Autodesk Inventor part; units mm, degrees
ref_plane "YZ Plane" through (0, 0, 0) normal (1, 0, 0) x (0, 1, 0)
ref_plane "XZ Plane" through (0, 0, 0) normal (0, 1, 0) x (-1, 0, 0)
ref_plane "XY Plane" through (0, 0, 0) normal (0, 0, 1) x (1, 0, 0)
sketch "Sketch1" plane through (0, 0, 0) normal (0, 0, 1) x (1, 0, 0)
  line L0 (-11.8297, 9.3175) -> (-7.8297, 9.3175)
  line L1 (-7.8297, 9.3175) -> (-7.8297, -24.6825)
  line L2 (-11.8297, -24.6825) -> (-11.8297, 9.3175)
  line L3 (16.1703, -24.6825) -> (16.1703, -28.6825)
  line L4 (16.1703, -28.6825) -> (-11.8297, -28.6825)
  line L5 (-11.8297, -28.6825) -> (-11.8297, -24.6825)
  line L6 (12.1703, -24.6825) -> (12.1703, 9.3175)
  line L7 (12.1703, 9.3175) -> (16.1703, 9.3175)
  line L8 (16.1703, 9.3175) -> (16.1703, -24.6825)
  line L9 (12.1703, -24.6825) -> (-7.8297, -24.6825)
  point P0 (0, 0)
  dimension "d0" = 4
  dimension "d1" = 34
  dimension "d5" = 4
  dimension "d6" = 4
  dimension "d7" = 34
  dimension "d14" = 24
  dimension "d15" = 28
  dimension "d16" = 38
  dimension "d18" = 9.3175
extrude "Extrusion1" add sketch "Sketch1" along normal blind 30
sketch "Sketch2" plane through (-11.8297, -28.6825, 0) normal (-1, 0, 0) x (0, 0, 1)
  line L0 (0, 0) -> (0, 38) construction
  line L1 (0, 0) -> (30, 0) construction
  line L2 (30, 38) -> (30, 0) construction
  line L3 (0, 38) -> (30, 38) construction
  line L4 (0, 38) -> (30, 38) construction
  line L5 (15, 38) -> (15, 0) construction
  circle A0 centre (15, 29.8727) radius 3.25
  point P0 (0, 28.6825)
  dimension "d10" = 6.5
extrude "Extrusion2" cut sketch "Sketch2" against normal through all
fillet "Fillet1" radius 10 4 edges at (-9.8297, 9.3175, 0) (14.1703, 9.3175, 0) (-9.8297, 9.3175, 30) (14.1703, 9.3175, 30)
sketch "Sketch3" plane through (-7.8297, -24.6825, 0) normal (0, 1, 0) x (1, 0, 0)
  line L0 (0, 0) -> (20, 0)
  line L1 (0, 0) -> (0, -30)
  line L2 (20, -30) -> (0, -30)
  line L3 (20, 0) -> (20, -30)
  circle A0 centre (10, -15) radius 4.25
  point P0 (7.8297, 0)
  dimension "d19" = 8.5
extrude "Extrusion3" cut sketch "Sketch3" against normal through all contours A0
fillet "Fillet2" radius 2 2 edges at (-7.8297, -24.6825, 15) (12.1703, -24.6825, 15)
equation "\"d1\" = d7"
properties part number "linear actuator bracket"
Check sheet for the modelled part. Datum: model origin and axes. Units: mm. A direction names the side the tool comes from. Give positions to 0.01 mm unless a question says otherwise; leave off trailing zeros. Loops run counter-clockwise (first coordinate to the right, second up) from the corner with the lowest first, then second, coordinate; pieces in that order, holes last. Notation, with made-up numbers: M -18,-25 L 24,-25 A18 cw 24,5 Z; hole C 33,80.25 d4. An arc over 180 degrees is marked long. Use a Markdown table: item, result. Add a question column.
Q1. Sectioned sample at D-D, the plane y = 3. Record the cut outline in (x, z).
Q2. Go/stop test with a flat-tipped pin: pin 1 (5 mm diameter, centred on y = 1.19, z = 15, fed in from -X). Record where the tip stops, or that it passes through.
Q3. Tool access check on faces 1 (the flat face through (-7.83, -6, 15)), 2 (the cylindrical face through (14.2, 6.47, 26.99)). Record the directions out of +Z, -Z, +X, -X, +Y, -Y that give a thin tool (end or side, any length) a straight path to the whole face; none if there is none.
Q4. Sectioned sample at C-C, the plane x = 0.5. Record the cut outline in (y, z), then the cut area to 3 significant figures.
Q5. Mould release check, pull along Z, two halves, no side actions. Record for faces 3 (the flat face through (2, -25, 30)), 4 (the cylindrical face through (14.2, 6.31, 2.85)), 5 (the cylindrical face through (-9.858, 1.333, 11.753)), 6 (the flat face through (5.5, -28.682, 18.1)): pulls with the +Z half, pulls with the -Z half, needs draft (parallel to the pull), parting line crosses it, or undercut.
Q6. Sectioned sample at B-B, the plane z = 15. Record the cut outline in (x, y), then the cut area to 3 significant figures.
Q7. Sectioned sample at A-A, the plane y = -12. Record the cut outline in (x, z).
Q8. Scan lines: line 1 along X through (y, z) = (6, 14.25); line 2 along X through (y, z) = (-26.45, 15); line 3 along Y through (x, z) = (13.05, 15). Record each from-to range of solid material in increasing order. Write a range as [from, to].
Verdict:
| question | item | result |
|---|---|---|
| 1 | outline | M -11.83,0.7 L -7.83,0.7 L -7.83,12.3 L -11.83,12.3 Z; M -11.83,17.7 L -7.83,17.7 L -7.83,29.3 L -11.83,29.3 Z; M 12.17,0.7 L 16.17,0.7 L 16.17,12.3 L 12.17,12.3 Z; M 12.17,17.7 L 16.17,17.7 L 16.17,29.3 L 12.17,29.3 Z |
| 2 | pin 1 | through |
| 3 | face 1 | +Z, -Z, +Y |
| 3 | face 2 | +Z, +X, -X, +Y |
| 4 | outline | M -28.68,0 L -24.68,0 L -24.68,11.09 L -28.68,11.09 Z; M -28.68,18.91 L -24.68,18.91 L -24.68,30 L -28.68,30 Z |
| 4 | area | 88.7 mm^2 |
| 5 | face 3 | pulls with the +Z half |
| 5 | face 4 | pulls with the -Z half |
| 5 | face 5 | undercut |
| 5 | face 6 | needs draft |
| 6 | outline | M -11.83,-28.68 L -2.08,-28.68 L -2.08,-24.68 L -5.83,-24.68 A2 cw -7.83,-22.68 L -7.83,-2.06 L -11.83,-2.06 Z; M -11.83,4.44 L -7.83,4.44 L -7.83,9.32 L -11.83,9.32 Z; M 6.42,-28.68 L 16.17,-28.68 L 16.17,-2.06 L 12.17,-2.06 L 12.17,-22.68 A2 cw 10.17,-24.68 L 6.42,-24.68 Z; M 12.17,4.44 L 16.17,4.44 L 16.17,9.32 L 12.17,9.32 Z |
| 6 | area | 300 mm^2 |
| 7 | outline | M -11.83,0 L -7.83,0 L -7.83,30 L -11.83,30 Z; M 12.17,0 L 16.17,0 L 16.17,30 L 12.17,30 Z |
| 8 | line 1 | [-11.83, -7.83], [12.17, 16.17] |
| 8 | line 2 | [-11.83, -2.08], [6.42, 16.17] |
| 8 | line 3 | [-28.68, -2.06], [4.44, 9.32] |
